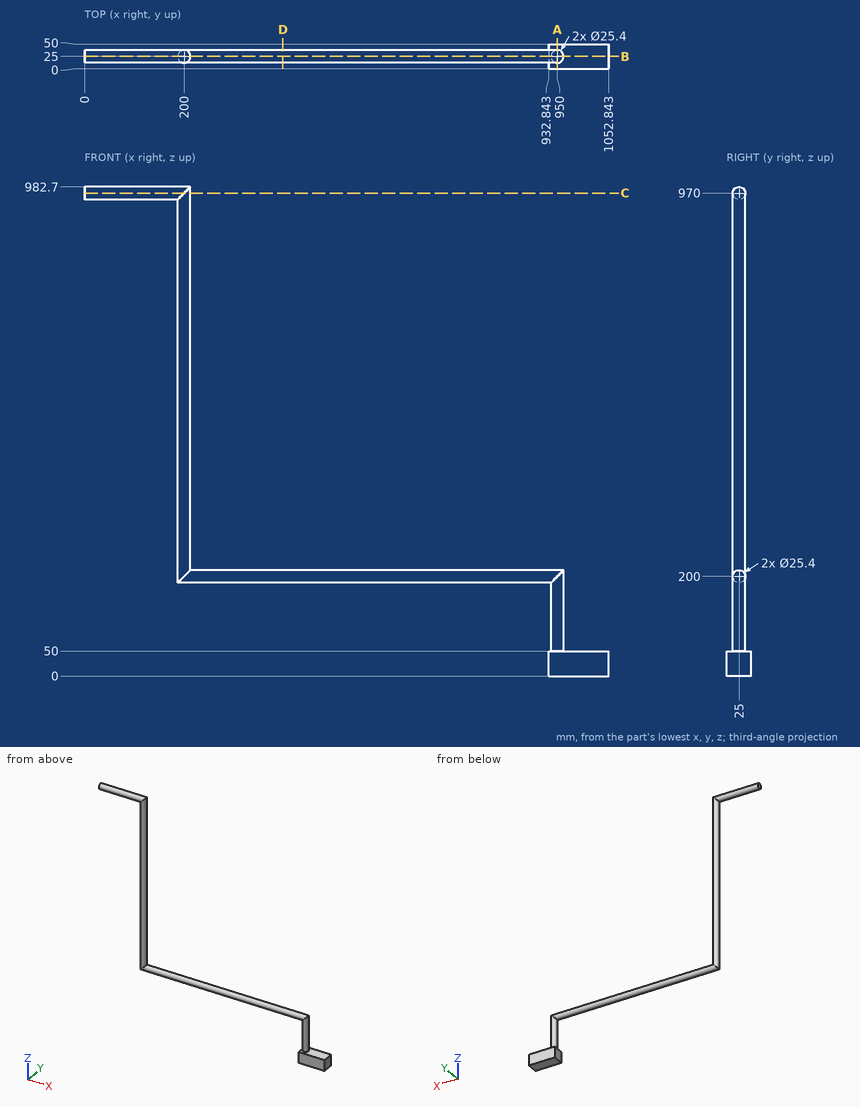
Design review of the part shown in the three views and the two pictorial views. Dimensions are in mm from the part's minimum x, y and z. Round coordinates to 2 decimals unless told otherwise and drop trailing zeros. Loops run counter-clockwise (first coordinate to the right, second up) from the corner with the lowest first, then second, coordinate; pieces in that order, holes last. Notation, with made-up numbers: M 32,-25 L 78,-25 A25 cw 78,8 Z; hole C -12,-37 d1. An arc over 180 degrees is marked long. Answer as a JSON object with one key per item and string values.
Item 1: We need section A-A on x = 950. Give the boundary of the cut face in (y, z).
Answer sheet:
{"outline": "M 0,0 L 50,0 L 50,50 L 37.7,50 L 37.7,200 A12.7 ccw 12.3,200 L 12.3,50 L 0,50 Z"}
Item 2: Clearance check with flat-ended pins moving along their axes: P1, Ø4, axis at y = 27.5, z = 391, coming from the +X side; P2, Ø6, axis at x = 547.5, z = 216.5, coming from the -Y side; P3, Ø3, axis at y = 30.5, z = 135, coming from the +X side; P4, Ø3, axis at x = 259, y = 30.5, coming from the +Z side. State where each tip first meets the part, or that it passes through.
Answer sheet:
{"P1": "stops at x = 212.69", "P2": "passes through", "P3": "stops at x = 962.05", "P4": "stops at z = 212.05"}
Item 3: Wall thickness on L1, parallel to X at y = 27, z = 226; L2, parallel to Z at x = 994.5, y = 39; L3, parallel to X at y = 26, z = 862: over which ranges is each line inside the solid? List them lowest first. Write a range as from..to.
Answer sheet:
{"L1": "x = 187.46..212.54", "L2": "z = 0..50", "L3": "x = 187.34..212.66"}
Item 4: We need section D-D on x = 398.5. Give the boundary of the cut face in (y, z).
Answer sheet:
{"outline": "C 25,200 d25.4"}
Item 5: We need section C-C on z = 970. Give the boundary of the cut face in (x, y).
Answer sheet:
{"outline": "M 0,12.3 L 200,12.3 A12.7 ccw 200,37.7 L 0,37.7 Z"}
Item 6: We need section B-B on y = 25. Give the boundary of the cut face in (x, z).
Answer sheet:
{"outline": "M 0,957.3 L 187.3,957.3 L 187.3,187.3 L 937.3,187.3 L 937.3,50 L 932.84,50 L 932.84,0 L 1052.84,0 L 1052.84,50 L 962.7,50 L 962.7,212.7 L 212.7,212.7 L 212.7,982.7 L 0,982.7 Z"}
